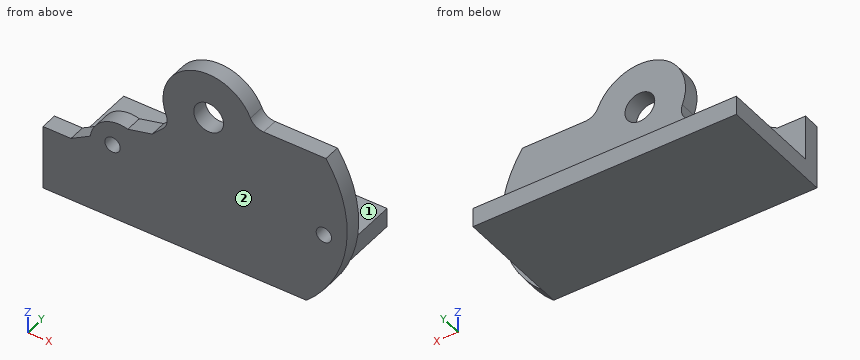
from build123d import *
from build123d.topology import SkipClean

# Parameters (mm, degrees)
CROQUIS1_W              = 70
CROQUIS1_H              = 65
EXTRUIR1_DEPTH          = 3.5
CROQUIS2_R              = 3.1
EXTRUIR2_DEPTH          = 5
EXTRUIR3_DEPTH          = 10
CROQUIS4_OUTSIDE_W      = 91.294
CROQUIS4_OUTSIDE_H      = 86.294
EXTRUIR4_DEPTH          = 10
REDONDEO1_R             = 3
EXTRUIR5_DEPTH          = 13.5
EXTRUIR6_DEPTH          = 3.5
CROQUIS7_R              = 1.6
EXTRUIR7_DEPTH          = 47.982330447
CROQUIS8_R              = 3.1
EXTRUIR8_DEPTH          = 5
CROQUIS9_W              = 0.7
CROQUIS9_H              = 10.5
EXTRUIR9_DEPTH          = 10
EXTRUIR10_DEPTH         = 63.752948337
EXTRUIR10_DEPTH_BACK    = 10
CROQUIS10_W             = 3.0625
CROQUIS10_H             = 5
CROQUIS11_W             = 54.8364
CROQUIS11_H             = 21.05596306
SALIENTE_EXTRUIR1_DEPTH = 4


with BuildPart() as part:
    # Croquis1 → Extruir1 (new body)
    with BuildSketch(Plane(origin=(0, 0, 0), x_dir=(1, 0, 0), z_dir=(0, 1, 0))):
        Rectangle(CROQUIS1_W, CROQUIS1_H)
    extrude(amount=EXTRUIR1_DEPTH)

    # Croquis2 → Extruir2 (cut)
    with BuildSketch(Plane(origin=(0, 3.5, 0), x_dir=(1, 0, 0), z_dir=(0, 1, 0))):
        with Locations(Location((0, -17.5, 0), (0, 0, 270))):
            Circle(CROQUIS2_R)
    extrude(amount=-EXTRUIR2_DEPTH, mode=Mode.SUBTRACT)

    # Croquis3 → Extruir3 (add)
    with BuildSketch(Plane(origin=(0, 3.5, 0), x_dir=(1, 0, 0), z_dir=(0, 1, 0))):
        with BuildLine():
            Line((-34.4868, 13.5), (20.3496, 13.5))
            Line((20.3496, 13.5), (20.3496, 0))
            Line((20.3496, 0), (17.146428199, 0))
            ThreePointArc((17.146428199, 0), (22.955777517, -8.939493087), (24.418230894, -19.5))
            Line((24.418230894, -19.5), (9.287087811, -19.5))
            ThreePointArc((9.287087811, -19.5), (-3.635492607, -26.276855559), (-7.981176331, -12.347250794))
            Line((-7.981176331, -12.347250794), (-18.680510212, -1.647916913))
            ThreePointArc((-18.680510212, -1.647916913), (-17.932408832, -0.806327142), (-17.146428199, 0))
            Line((-17.146428199, 0), (-34.4868, 0))
            Line((-34.4868, 0), (-34.4868, 13.5))
        make_face()
        with BuildLine():
            Line((-32.9868, 1.5), (-12.961481397, 1.5))
            ThreePointArc((-12.961481397, 1.5), (-14.868021343, 0.048274597), (-16.613165932, -1.593940849))
            Line((-16.613165932, -1.593940849), (-5.999348286, -12.207758495))
            ThreePointArc((-5.999348286, -12.207758495), (-3.061467459, -24.89103626), (7.984359711, -18))
            Line((7.984359711, -18), (22.994564575, -18))
            ThreePointArc((22.994564575, -18), (20.451694563, -6.977253708), (12.961481397, 1.5))
            Line((12.961481397, 1.5), (18.8496, 1.5))
            Line((18.8496, 1.5), (18.8496, 12))
            Line((18.8496, 12), (-32.9868, 12))
            Line((-32.9868, 12), (-32.9868, 1.5))
        make_face(mode=Mode.SUBTRACT)
    extrude(amount=EXTRUIR3_DEPTH)

    # Croquis4 outside → Extruir4 (cut)
    with SkipClean():  # the faces are left unmerged after this step: merging them gives an invalid solid
        with BuildSketch(Plane(origin=(0, 3.5, 0), x_dir=(1, 0, 0), z_dir=(0, 1, 0))):
            Rectangle(CROQUIS4_OUTSIDE_W, CROQUIS4_OUTSIDE_H)
            with BuildLine():
                Line((-34.4868, 0), (-17.146428199, 0))
                ThreePointArc((-17.146428199, 0), (-17.932408832, -0.806327142), (-18.680510212, -1.647916913))
                Line((-18.680510212, -1.647916913), (-7.981176331, -12.347250794))
                ThreePointArc((-7.981176331, -12.347250794), (-3.635492607, -26.276855559), (9.287087811, -19.5))
                Line((9.287087811, -19.5), (24.418230894, -19.5))
                ThreePointArc((24.418230894, -19.5), (22.955777517, -8.939493087), (17.146428199, 0))
                Line((17.146428199, 0), (20.3496, 0))
                Line((20.3496, 0), (20.3496, 13.5))
                Line((20.3496, 13.5), (-34.4868, 13.5))
                Line((-34.4868, 13.5), (-34.4868, 0))
            make_face(mode=Mode.SUBTRACT)
        extrude(amount=-EXTRUIR4_DEPTH, mode=Mode.SUBTRACT)

    # Redondeo1
    redondeo1_edges = [part.edges().sort_by_distance(p)[0] for p in [
        (-7.981176331, 8.5, 12.347250794),
        (9.287087811, 8.5, 19.5),
        (-5.999348286, 8.5, 12.207758495),
        (7.984359711, 8.5, 18),
    ]]
    fillet(redondeo1_edges, radius=REDONDEO1_R)

    # Croquis5 → Extruir5 (add)
    with SkipClean():  # the faces are left unmerged after this step: merging them gives an invalid solid
        with BuildSketch(Plane.XZ):
            with BuildLine():
                Line((-18.680510212, 1.647916913), (-14.437869525, 5.8905576))
                ThreePointArc((-14.437869525, 5.8905576), (-21.723092903, 6.819250451), (-24.449770984, 0))
                Line((-24.449770984, 0), (-17.146428199, 0))
                ThreePointArc((-17.146428199, 0), (-17.932408832, 0.806327142), (-18.680510212, 1.647916913))
            make_face()
            with BuildLine():
                Line((20.3496, 0), (20.3496, -13.5))
                ThreePointArc((20.3496, -13.5), (28.665212431, 2.225567304), (24.418230894, 19.5))
                ThreePointArc((24.418230894, 19.5), (22.955777517, 8.939493087), (17.146428199, 0))
                Line((17.146428199, 0), (20.3496, 0))
            make_face()
        extrude(amount=-EXTRUIR5_DEPTH)

    # Chaflán1
    # the kernel refuses this chamfer: 5, 4.044665138 mm, written as the material it adds along each edge
    with BuildSketch(Plane(origin=(-14.437869525, 3.5, 5.8905576), x_dir=(-0.8528028654224412, 0, 0.5222329678670944), z_dir=(0, 1, 0))) as chafl_n1_piece_1:
        with BuildLine():
            Line((2.946399951, -0.141421356), (-1.029187491, 3.834166086))
            Line((-1.029187491, 3.834166086), (-1.126417207, 3.810791264))
            ThreePointArc((-1.126417207, 3.810791264), (-0.561046898, 1.905915324), (-0.097229716, -0.023374822))
            Line((-0.097229716, -0.023374822), (0.023374822, -0.097229716))
            ThreePointArc((0.023374822, -0.097229716), (1.474874577, 0.065772974), (2.923025129, -0.238651072))
            Line((2.923025129, -0.238651072), (2.946399951, -0.141421356))
        make_face()
    extrude(amount=10)
    with BuildSketch(Plane(origin=(-24.449770984, 3.5, 0), x_dir=(-0.08263556343231732, 0, 0.9965798330571533), z_dir=(0, 1, 0))) as chafl_n1_piece_2:
        with BuildLine():
            Line((2.416506842, 0.180832589), (0.262590721, -4.378032196))
            Line((0.262590721, -4.378032196), (0.162932738, -4.386295752))
            ThreePointArc((0.162932738, -4.386295752), (0.081510488, -2.193144218), (-0.099657983, -0.008263556))
            Line((-0.099657983, -0.008263556), (0.019425577, 0.098095091))
            ThreePointArc((0.019425577, 0.098095091), (1.209024094, -0.014134236), (2.397081265, 0.278927681))
            Line((2.397081265, 0.278927681), (2.416506842, 0.180832589))
        make_face()
    extrude(amount=10)
    with BuildSketch(Plane(origin=(-24.449770984, 0, 0), x_dir=(-1, 0, 0), z_dir=(0, 1, 0))) as chafl_n1_piece_3:
        with BuildLine():
            Line((4.384757927, -0.10008854), (0.019475293, 2.423185189))
            Line((0.019475293, 2.423185189), (-0.079889541, 2.411932193))
            ThreePointArc((-0.079889541, 2.411932193), (0.113994282, 1.203721039), (-0.096154346, 0.027465282))
            Line((-0.096154346, 0.027465282), (0, -0.1))
            ThreePointArc((0, -0.1), (2.192378963, -0.1), (4.384757927, -0.20008854))
            Line((4.384757927, -0.20008854), (4.384757927, -0.10008854))
        make_face()
    extrude(amount=3.5)
    with BuildSketch(Plane(origin=(-14.437869525, 0, 5.8905576), x_dir=(0.7071067811865478, 0, 0.7071067811865472), z_dir=(0, 1, 0))) as chafl_n1_piece_4:
        with BuildLine():
            Line((3.968519544, 0.104446594), (-0.826219316, -2.831719321))
            Line((-0.826219316, -2.831719321), (-0.91529167, -2.786264775))
            ThreePointArc((-0.91529167, -2.786264775), (-0.280798425, -1.449390681), (-0.1, 0))
            Line((-0.1, 0), (0, 0.1))
            ThreePointArc((0, 0.1), (1.984259772, 0.1), (3.968519544, 0.204446594))
            Line((3.968519544, 0.204446594), (3.968519544, 0.104446594))
        make_face()
    extrude(amount=3.5)


with BuildPart() as body_2:
    # Croquis6 → Extruir6 (new body)
    with BuildSketch(Plane(origin=(0, 13.5, 0), x_dir=(1, 0, 0), z_dir=(0, 1, 0))):
        with BuildLine():
            Line((-34.4868, 13.5), (-34.4868, 0))
            Line((-34.4868, 0), (-28.661374979, 0))
            Line((-28.661374979, 0), (-24.642400208, -2.323096648))
            ThreePointArc((-24.642400208, -2.323096648), (-21.929637735, -6.692039268), (-16.829963308, -7.355409896))
            Line((-16.829963308, -7.355409896), (-11.752306982, -8.576120143))
            Line((-11.752306982, -8.576120143), (-9.515139435, -10.813287689))
            ThreePointArc((-9.515139435, -10.813287689), (-8.69974084, -12.321679102), (-8.843709432, -14.030302105))
            ThreePointArc((-8.843709432, -14.030302105), (-3.635492607, -26.276855559), (8.70689382, -21.3))
            ThreePointArc((8.70689382, -21.3), (9.813271565, -19.99001992), (11.456439237, -19.5))
            Line((11.456439237, -19.5), (24.418230894, -19.5))
            ThreePointArc((24.418230894, -19.5), (28.665212431, -2.225567304), (20.3496, 13.5))
            Line((20.3496, 13.5), (-34.4868, 13.5))
        make_face()
    extrude(amount=EXTRUIR6_DEPTH)


with BuildPart() as extruir7_tool:
    # Croquis7 → Extruir7 (new, through all)
    with BuildSketch(Plane(origin=(0, 17, 0), x_dir=(1, 0, 0), z_dir=(0, 1, 0))):
        with Locations(Location((-20, -2.5, 0), (0, 0, 270))):
            Circle(CROQUIS7_R)
        with Locations(Location((24, -2.5, 0), (0, 0, 270))):
            Circle(CROQUIS7_R)
    extrude(amount=-EXTRUIR7_DEPTH)


with BuildPart() as part_1:
    add(part.part)

    # Extruir7: cut by extruir7_tool
    add(extruir7_tool.part, mode=Mode.SUBTRACT)

    # Croquis9 → Extruir9 (cut)
    with BuildSketch(Plane(origin=(0, 13.5, 0), x_dir=(1, 0, 0), z_dir=(0, 1, 0))):
        with Locations((19.1996, 6.75)):
            Rectangle(CROQUIS9_W, CROQUIS9_H)
    extrude(amount=-EXTRUIR9_DEPTH, mode=Mode.SUBTRACT)

    # Croquis10 → Extruir10 (cut, two sides: drawn at the far end of the back side and taken through both)
    with BuildSketch(Plane.ZY.offset(-19.5496).offset(-EXTRUIR10_DEPTH_BACK)):
        with Locations((-8.9375, 8.5)):
            Rectangle(CROQUIS10_W, CROQUIS10_H)
    extrude(amount=EXTRUIR10_DEPTH + EXTRUIR10_DEPTH_BACK, mode=Mode.SUBTRACT)


with BuildPart() as body_2_1:
    add(body_2.part)

    # Extruir7: cut by extruir7_tool
    add(extruir7_tool.part, mode=Mode.SUBTRACT)

    # Croquis8 → Extruir8 (cut)
    with BuildSketch(Plane(origin=(0, 17, 0), x_dir=(1, 0, 0), z_dir=(0, 1, 0))):
        with Locations(Location((0, -17.5, 0), (0, 0, 270))):
            Circle(CROQUIS8_R)
    extrude(amount=-EXTRUIR8_DEPTH, mode=Mode.SUBTRACT)

    # Croquis11 → Saliente-Extruir1 (add)
    with BuildSketch(Plane(origin=(0, 0, -13.5), x_dir=(-1, 0, 0), z_dir=(0, 0, -1))):
        with Locations((7.0686, 27.52798153)):
            Rectangle(CROQUIS11_W, CROQUIS11_H)
    extrude(amount=-SALIENTE_EXTRUIR1_DEPTH)


solid = body_2_1.part
Input: part model. Units: mm. Frame: model coordinates. Face numbers are marked on the shaded views. A direction names the side the tool comes from. Round coordinates to 2 decimals unless told otherwise and drop trailing zeros. Loops run counter-clockwise (first coordinate to the right, second up) from the corner with the lowest first, then second, coordinate; pieces in that order, holes last. Notation, with made-up numbers: M 56,4.25 L 82,4.25 A33 cw 82,36.25 Z; hole C 75,23 d7. An arc over 180 degrees is marked long. Answer as CSV lines item,"result". Start each with the question number.
(1) Section B-B, the plane x = 16. Output: boundary loops of the cut face in (y, z).
(2) Section D-D, the plane y = 15.75. Output: boundary loops of the cut face in (x, z).
(3) Section C-C, the plane z = 17.5. Output: boundary loops of the cut face in (x, y), plus the area to 3 significant figures.
(4) Section A-A, the plane x = 0. Output: boundary loops of the cut face in (y, z), plus the area to 3 significant figures.
(5) Line query: line 1 (X direction, y = 15.2, z = 2.5); line 2 (Y direction, x = -13, z = -6); line 3 (Z direction, x = -23, y = 29.75). Output: solid intervals per line, ascending. Write a range as [from, to].
(6) First-contact query: pin 1 (8 mm diameter, centred on x = -19, z = -7, fed in from +Y); pin 2 (8 mm diameter, centred on x = -8, z = 4.5, fed in from +Y); pin 3 (4.5 mm diameter, centred on y = 31, z = -11, fed in from +X); pin 4 (3 mm diameter, centred on x = 16, y = 16, fed in from +Z). Flat tips, straight axial feed; report the tip coordinate or a pass-through.
(7) Reachability of the marked faces 1 and 2 from +Z, -Z, +X, -X, +Y, -Y: full face, straight path, thin tool, end or side. Return the list, or none.
Values found:
1,outline,"M 13.5,-13.5 L 38.06,-13.5 L 38.06,-9.5 L 17,-9.5 L 17,19.5 L 13.5,19.5 Z"
2,outline,"M -34.49,-13.5 L 20.35,-13.5 A25 ccw 24.42,19.5 L 11.46,19.5 A3 cw 8.71,21.3 A9.5 ccw -8.84,14.03 A3 cw -9.52,10.81 L -11.75,8.58 L -16.83,7.36 A6 ccw -24.64,2.32 L -28.66,0 L -34.49,0 Z; hole C -20,2.5 d3.2; hole C 0,17.5 d6.2; hole C 24,2.5 d3.2"
3,outline,"M -9.5,13.5 L -3.1,13.5 L -3.1,17 L -9.5,17 Z; M 3.1,13.5 L 25.67,13.5 L 25.67,17 L 3.1,17 Z"
3,area,"101 mm²"
4,outline,"M 13.5,-13.5 L 38.06,-13.5 L 38.06,-9.5 L 17,-9.5 L 17,14.4 L 13.5,14.4 Z; M 13.5,20.6 L 17,20.6 L 17,27 L 13.5,27 Z"
4,area,"204 mm²"
5,line 1,"x = [-24.62, -21.6], [-18.4, 22.4], [25.6, 28.7]"
5,line 2,"y = [13.5, 17]"
5,line 3,"z = [-13.5, -9.5]"
6,pin 1,"stops at y = 38.06"
6,pin 2,"stops at y = 17"
6,pin 3,"stops at x = 20.35"
6,pin 4,"stops at z = 19.5"
7,face 1,"+Z, +X, -X, +Y"
7,face 2,"+Z, -Z, +X, -X, -Y"
